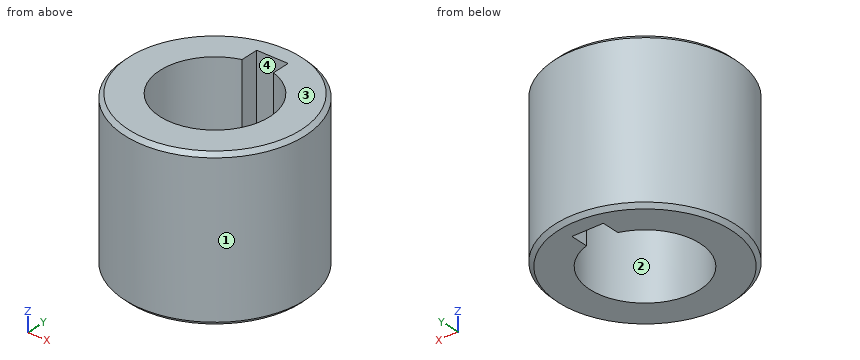
```python
from build123d import *

# Parameters (mm, degrees)
F0_R     = 23
F0_R_2   = 14.03
F1_DEPTH = 40
F3_DEPTH = 40.001
F4_SIZE  = 1


with BuildPart() as f1:
    # F0 (on Top) → F1 (new body)
    with BuildSketch(Plane.XY):
        Circle(F0_R)
        Circle(F0_R_2, mode=Mode.SUBTRACT)
    extrude(amount=F1_DEPTH)

    # F2 (on face) → F3 (cut, through all)
    with BuildSketch(Plane.XY.offset(40)):
        with BuildLine():
            Line((4, 13.44771), (4, 18.03))
            Line((4, 18.03), (-4, 18.03))
            Line((-4, 18.03), (-4, 13.44771))
            ThreePointArc((-4, 13.44771), (0, 14.03), (4, 13.44771))
        make_face()
    extrude(amount=-F3_DEPTH, mode=Mode.SUBTRACT)

    # F4
    f4_edges = [f1.edges().sort_by_distance(p)[0] for p in [
        (-23, 0, 40),
        (-23, 0, 0),
    ]]
    chamfer(f4_edges, length=F4_SIZE)


solid = f1.part
```
The model under review builds one solid part; all positions refer to its coordinate system, in mm. Face numbers are marked on the shaded views. Round coordinates to 2 decimals unless told otherwise and drop trailing zeros. Loops run counter-clockwise (first coordinate to the right, second up) from the corner with the lowest first, then second, coordinate; pieces in that order, holes last.
Item 1: Clearance check with flat-ended pins moving along their axes: pin 1 Ø5 at (y, z) = (-8.5, 35.5) entering from +X; pin 2 Ø12 at (x, y) = (-18, 16.5) entering from -Z; pin 3 Ø6 at (x, z) = (-17.5, 9) entering from +Y; pin 4 Ø1 at (y, z) = (12.5, 13) entering from +X. State where each tip first meets the part, or that it passes through.
Determined:
pin 1: stops at x = 22.2
pin 2: stops at z = 0
pin 3: stops at y = 17.85
pin 4: stops at x = 19.62
Item 2: Take a section at B-B (x = 0). Write out the cut boundary in (y, z).
Determined:
outline: (-23, 1) - (-22, 0) - (-14.03, 0) - (-14.03, 40) - (-22, 40) - (-23, 39) - close; (18.03, 0) - (22, 0) - (23, 1) - (23, 39) - (22, 40) - (18.03, 40) - close
Item 3: Take a section at C-C (z = 19.5). Write out the cut boundary in (x, y), then the cut area to 3 significant figures.
Determined:
outline: circle Ø46 at (0, 0); hole (-4, 13.45) arc R14.03 ccw (long way) to (4, 13.45) - (4, 18.03) - (-4, 18.03) - close
area: 1,010 mm2
Item 4: For line 1 (Y direction, x = 0, z = 17); line 2 (Y direction, x = -7.5, z = 26.5); line 3 (X direction, y = 1, z = 13.5), list the stretches that pass through material, from the lowest coordinate up.
Determined:
line 1: y = -23 to -14.03, 18.03 to 23
line 2: y = -21.74 to -11.86, 11.86 to 21.74
line 3: x = -22.98 to -13.99, 13.99 to 22.98
Item 5: Take a section at A-A (y = 0). Write out the cut boundary in (x, z).
Determined:
outline: (-23, 1) - (-22, 0) - (-14.03, 0) - (-14.03, 40) - (-22, 40) - (-23, 39) - close; (14.03, 0) - (22, 0) - (23, 1) - (23, 39) - (22, 40) - (14.03, 40) - close
Item 6: Mouldability with a two-part tool opening along X and no side actions: class the marked faces 1, 2, 3 and 4 as released by +X, released by -X, zero draft, split by the parting line, or undercut.
Determined:
face 1: split by the parting line
face 2: undercut
face 3: zero draft
face 4: undercut
